Geometry: see drawing. Coordinates: mm, zero at the bounding-box minimum. A direction names the side the tool comes from. Round coordinates to 2 decimals unless told otherwise and drop trailing zeros. Loops run counter-clockwise (first coordinate to the right, second up) from the corner with the lowest first, then second, coordinate; pieces in that order, holes last. Notation, with made-up numbers: (-27, -28.5) - (21, -28.5) arc R27 cw to (21, -12.5) - close; hole circle Ø3 at (67, 31.25). An arc over 180 degrees is marked (long way). Write item = value, one per line. Start each with the question number.
Item 1: Section B-B (z = 165). Return loops of the section in (x, y).
Item 2: Draft query along X for the marked faces 4, 5 and 6. Return one class per face: pulls with the +X half, pulls with the -X half, needs draft (parallel to the pull), parting line crosses it, or undercut.
Item 3: First-contact query: pin 1 (24 mm diameter, centred on x = 218, z = 61, fed in from +Y). Flat tip, straight axial feed; report the tip coordinate or a pass-through.
Item 4: Section A-A (y = 79.5). Return loops of the section in (x, z).
Item 5: Section D-D (z = 60). Return loops of the section in (x, y), plus the area to 3 significant figures.
Item 6: Section C-C (x = 140). Return loops of the section in (y, z).
Item 7: Access query for the marked faces 1, 2 and 3. Directions: +Z, -Z, +X, -X, +Y, -Y. A direction counts if a zero-diameter tool reaches every point of the face in a straight line with its end or side. Return the directions, or none.
Item 8: Line query: line 1 (X direction, y = 115, z = 165); line 2 (X direction, y = 117.5, z = 60); line 3 (Y direction, x = 30, z = 201.5). Output: solid intervals per line, ascending. Write a range as from..to.
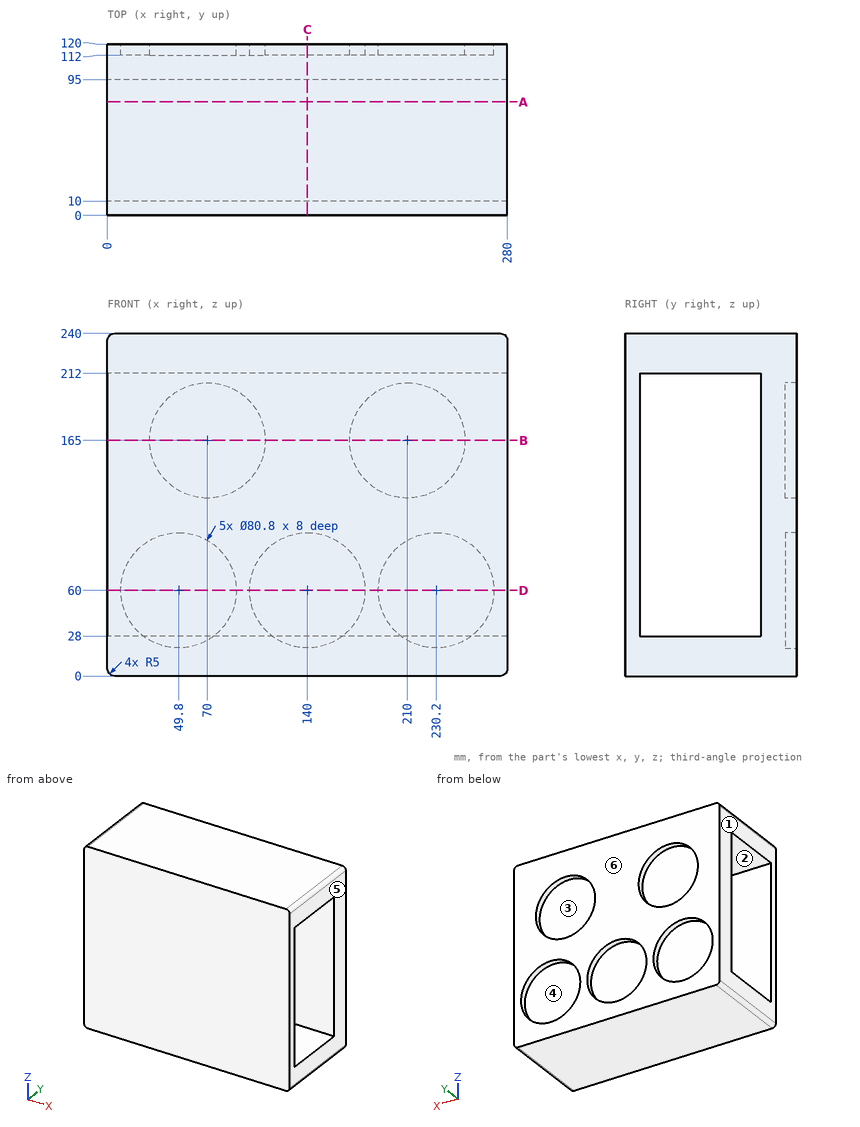
Taken from the geometry:
q1.outline = (0, 0) - (280, 0) - (280, 10) - (0, 10) - close; (0, 95) - (280, 95) - (280, 120) - (250.4, 120) - (250.4, 112) - (169.6, 112) - (169.6, 120) - (110.4, 120) - (110.4, 112) - (29.6, 112) - (29.6, 120) - (0, 120) - close
q2.face_4 = undercut
q2.face_5 = pulls with the +X half
q2.face_6 = needs draft
q3.pin_1 = 112
q4.outline = (0, 5) arc R5 ccw to (5, 0) - (275, 0) arc R5 ccw to (280, 5) - (280, 28) - (0, 28) - close; (0, 212) - (280, 212) - (280, 235) arc R5 ccw to (275, 240) - (5, 240) arc R5 ccw to (0, 235) - close
q5.outline = (0, 0) - (280, 0) - (280, 10) - (0, 10) - close; (0, 95) - (280, 95) - (280, 120) - (270.6, 120) - (270.6, 112) - (189.8, 112) - (189.8, 120) - (180.4, 120) - (180.4, 112) - (99.6, 112) - (99.6, 120) - (90.2, 120) - (90.2, 112) - (9.4, 112) - (9.4, 120) - (0, 120) - close
q5.area = 7,860 mm^2
q6.outline = (0, 0) - (120, 0) - (120, 19.6) - (112, 19.6) - (112, 100.4) - (120, 100.4) - (120, 240) - (0, 240) - close; hole (10, 28) - (95, 28) - (95, 212) - (10, 212) - close
q7.face_1 = +Z, -Z, -X, +Y, -Y
q7.face_2 = +X, -X
q7.face_3 = +Y
q8.line_1 = 0..29.6, 110.4..169.6, 250.4..280
q8.line_2 = 0..9.4, 90.2..99.6, 180.4..189.8, 270.6..280
q8.line_3 = 0..10, 95..120
